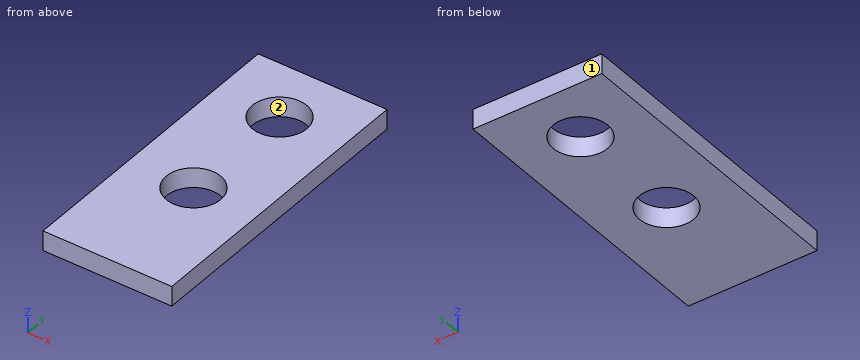
```python
from build123d import *

# Parameters (mm, degrees)
F1_DEPTH = 82.55
F2_R     = 17.4625
F3_DEPTH = 25.4
F4_W     = 82.55
F4_H     = 114.3
F5_DEPTH = 25.401


with BuildPart() as f1:
    # F0 (on Right) → F1 (new body)
    with BuildSketch(Plane.YZ):
        Polygon((0, 127), (0, 0), (190.5, 0), (190.5, 12.7), (25.4, 12.7), (25.4, 127), align=None)
    extrude(amount=F1_DEPTH)

    # F2 (on face) → F3 (cut)
    with BuildSketch(Plane.XY.offset(12.7)):
        with Locations((41.275, 76.2)):
            Circle(F2_R)
        with Locations((41.275, 152.4)):
            Circle(F2_R)
    extrude(amount=-F3_DEPTH, mode=Mode.SUBTRACT)

    # F4 (on face) → F5 (cut, through all)
    with BuildSketch(Plane(origin=(0, 25.4, 0), x_dir=(-1, 0, 0), z_dir=(0, 1, 0))):
        with Locations((-41.275, 69.85)):
            Rectangle(F4_W, F4_H)
    extrude(amount=-F5_DEPTH, mode=Mode.SUBTRACT)


solid = f1.part
```
Read the model definition and answer for the solid it produces. Units are mm, in the model's axes. Face numbers are marked on the shaded views. Give positions to 0.01 mm unless a question says otherwise; leave off trailing zeros. Loops run counter-clockwise (first coordinate to the right, second up) from the corner with the lowest first, then second, coordinate; pieces in that order, holes last.
Item 1: The part is cut by section D-D (x = 40). Write down the section's boundary in (y, z), and give its area (3 significant figures).
Item 2: The mould has two halves that part along X. Classify the marked faces 1 and 2: released by +X, released by -X, zero draft, split by the parting line, or undercut.
Item 3: The part is cut by section B-B (z = 9.5). Give the number of separate pieces and of enclosed holes in the cut face, and give its area (3 significant figures).
Item 4: Each of these flat-tipped pins is pushed along its axis until it touches: pin 1 Ø1.5 at (x, z) = (17, 7.5) entering from -Y; pin 2 Ø21 at (x, y) = (41.275, 152.4) entering from -Z. Where does it stop, or does it pass through?
Item 5: The part is cut by section A-A (y = 76.2). Write down the section's boundary in (x, z).
Item 6: The part is cut by section C-C (x = 27). Write down the section's boundary in (y, z).
Item 7: Find the intervals of material crossed by line 1 along Y through (x, z) = (41, 3.75); line 2 along Y through (x, z) = (32, 2.75); line 3 along X through (y, z) = (156, 8.75), in increasing order.
Taken from the geometry:
1. outline: (0, 0) - (58.78, 0) - (58.78, 12.7) - (0, 12.7) - close; (93.62, 0) - (134.98, 0) - (134.98, 12.7) - (93.62, 12.7) - close; (169.82, 0) - (190.5, 0) - (190.5, 12.7) - (169.82, 12.7) - close
1. area: 1,530 mm2
2. face 1: zero draft
2. face 2: undercut
3. separate pieces: 1
3. enclosed holes: 2
3. area: 13,800 mm2
4. pin 1: stops at y = 0
4. pin 2: passes through
5. outline: (0, 0) - (23.81, 0) - (23.81, 12.7) - (0, 12.7) - close; (58.74, 0) - (82.55, 0) - (82.55, 12.7) - (58.74, 12.7) - close
6. outline: (0, 0) - (66.14, 0) - (66.14, 12.7) - (0, 12.7) - close; (86.26, 0) - (142.34, 0) - (142.34, 12.7) - (86.26, 12.7) - close; (162.46, 0) - (190.5, 0) - (190.5, 12.7) - (162.46, 12.7) - close
7. line 1: y = 0 to 58.74, 93.66 to 134.94, 169.86 to 190.5
7. line 2: y = 0 to 61.4, 91 to 137.6, 167.2 to 190.5
7. line 3: x = 0 to 24.19, 58.36 to 82.55
